Here's the drawing with two shaded views (mm, measured from the low corner). I have some questions. Give positions to 0.01 mm unless a question says otherwise; leave off trailing zeros. Write each loop counter-clockwise with the first axis right and the second up, starting at its lowest first coordinate (ties: lowest second). Pieces come first, ordered by that corner, then holes.
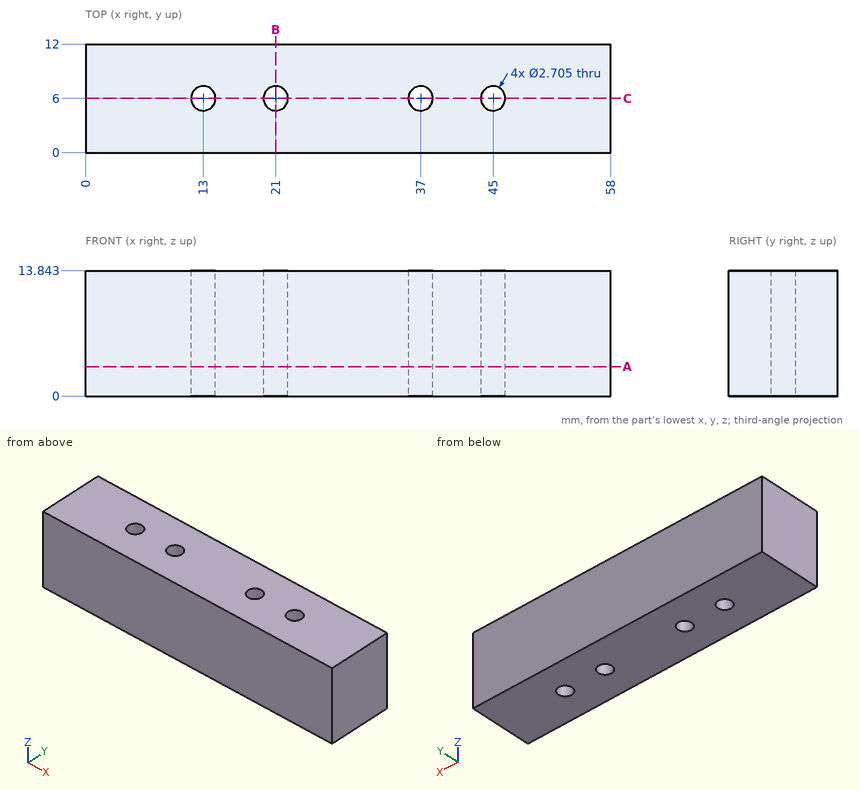
1) Please list where these lines run through material, in increasing order: L1, parallel to Y at x = 13, z = 7; L2, parallel to X at y = 5.25, z = 10; L3, parallel to X at y = 5, z = 8.
Values follow:
L1: y = 0 to 4.65, 7.35 to 12
L2: x = 0 to 11.87, 14.13 to 19.87, 22.13 to 35.87, 38.13 to 43.87, 46.13 to 58
L3: x = 0 to 12.09, 13.91 to 20.09, 21.91 to 36.09, 37.91 to 44.09, 45.91 to 58
2) Suppose I cut it at C-C on y = 6. Write out the boundary of the cut face in (x, z), plus the area to 3 significant figures.
Values follow:
outline: (0, 0) - (11.65, 0) - (11.65, 13.84) - (0, 13.84) - close; (14.35, 0) - (19.65, 0) - (19.65, 13.84) - (14.35, 13.84) - close; (22.35, 0) - (35.65, 0) - (35.65, 13.84) - (22.35, 13.84) - close; (38.35, 0) - (43.65, 0) - (43.65, 13.84) - (38.35, 13.84) - close; (46.35, 0) - (58, 0) - (58, 13.84) - (46.35, 13.84) - close
area: 653 mm2
3) Suppose I cut it at A-A on z = 3.25. Write out the boundary of the cut face in (x, y) (1 decimal).
Values follow:
outline: (0, 0) - (58, 0) - (58, 12) - (0, 12) - close; hole circle Ø2.7 at (13, 6); hole circle Ø2.7 at (21, 6); hole circle Ø2.7 at (37, 6); hole circle Ø2.7 at (45, 6)
4) Suppose I cut it at B-B on x = 21. Write out the boundary of the cut face in (y, z).
Values follow:
outline: (0, 0) - (4.65, 0) - (4.65, 13.84) - (0, 13.84) - close; (7.35, 0) - (12, 0) - (12, 13.84) - (7.35, 13.84) - close
